Here's how the part is built. I have some questions about the finished solid (model axes, mm). A direction names the side the tool comes from. Coordinates: 2 decimals unless noted, no trailing zeros. Write each loop counter-clockwise with the first axis right and the second up, starting at its lowest first coordinate (ties: lowest second). Pieces come first, ordered by that corner, then holes.
Item 1: If we section it at B-B (y = 6): Please give me the cut outline in (x, z) (3 decimals), then the cut area to 3 significant figures.
Item 2: If we section it at A-A (x = -10.5): Please give me the cut outline in (y, z) (3 decimals), then the cut area to 3 significant figures.
Item 3: If we section it at C-C (z = 1): Please give me the cut outline in (x, y), then the cut area to 3 significant figures.
Item 4: I'm going to push flat-ended pins straight in: pin 1 Ø3 at (x, z) = (-9.5, -4.5) entering from +Y; pin 2 Ø2 at (x, z) = (5, 3.5) entering from -Y; pin 3 Ø1.2 at (x, y) = (6.5, -14) entering from +Z; pin 4 Ø0.8 at (x, z) = (-1.5, 4) entering from +Y. Where does each tip first touch, or does it pass through?
Item 5: We'd pull the mould along X, two halves only. Please class faces 4 (the face through (15.77, 0, 0)), 5 (the face through (3.493, 12.808, -4.081)), 6 (the face through (-6.15, 1, 8)): +X half, -X half, draft (parallel to the pull), parting line (faces both ways), or undercut.
Item 6: If we section it at D-D (z = 3.75): Please give me the cut outline in (x, y).
Item 7: For faces 1 (the face through (0, -12.7, 4)), 2 (the face through (3.283, 14.174, 4.078)), 3 (the face through (12.8, 0, 0)), which set-ups out of +Z, -Z, +X, -X, +Y, -Y let a thin tool reach every point of the face, with its end or its side?
Item 8: If I drill on line 1 (X direction, y = -7, z = -2.5); line 2 (Z direction, x = -10, y = 3) (3 decimals); line 3 (Y direction, x = -0.5, z = 3), over which ranges is the centre line in solid material (lowest first)?
from build123d import *

# Parameters (mm, degrees)
ESQUISSE1_W             = 31.54
ESQUISSE1_H             = 30.3
BOSS_EXTRU_1_DEPTH      = 6.71
ESQUISSE2_W             = 12.3
ESQUISSE2_H             = 15.3
BOSS_EXTRU_2_DEPTH      = 3.6
ESQUISSE9_W             = 25.6
ESQUISSE9_H             = 10.95
ENL_V_MAT_EXTRU_2_DEPTH = 36.680232623
BOSS_EXTRU_3_START      = -5.3
BOSS_EXTRU_3_DEPTH      = 6
ENL_V_MAT_EXTRU_1_DEPTH = 3.4
ESQUISSE5_W             = 16
ESQUISSE5_H             = 8.3
BOSS_EXTRU_4_DEPTH      = 0.8
BOSS_EXTRU_5_DEPTH      = 0.05
ESQUISSE7_W             = 4.9
ESQUISSE7_H             = 4.9
BOSS_EXTRU_6_DEPTH      = 1.8
ESQUISSE8_R             = 2.575
BOSS_EXTRU_7_DEPTH      = 3.55
ESQUISSE10_W            = 7
ESQUISSE10_H            = 3.3
BOSS_EXTRU_8_DEPTH      = 2.45
ESQUISSE11_W            = 3
ESQUISSE11_H            = 1.48
BOSS_EXTRU_9_DEPTH      = 0.3


with BuildPart() as part:
    # Esquisse1 → Boss.-Extru.1 (new, symmetric)
    with BuildSketch(Plane.XY):
        Rectangle(ESQUISSE1_W, ESQUISSE1_H)
    extrude(amount=BOSS_EXTRU_1_DEPTH, both=True)

    # Esquisse2 → Boss.-Extru.2 (add)
    with BuildSketch(Plane.XY.offset(6.71)):
        with Locations((0, 0.9)):
            Rectangle(ESQUISSE2_W, ESQUISSE2_H)
    extrude(amount=BOSS_EXTRU_2_DEPTH)

    # Esquisse9 → Enlèv. mat.-Extru.2 (cut, through all)
    with BuildSketch(Plane(origin=(0, 15.15, 0), x_dir=(1, 0, 0), z_dir=(0, 1, 0))):
        Rectangle(ESQUISSE9_W, ESQUISSE9_H)
    extrude(amount=-ENL_V_MAT_EXTRU_2_DEPTH, mode=Mode.SUBTRACT)

    # Esquisse3 → Boss.-Extru.3 (add)
    with BuildSketch(Plane(origin=(0, 15.15, 0), x_dir=(1, 0, 0), z_dir=(0, 1, 0)).offset(BOSS_EXTRU_3_START)):
        Polygon((-4, -2.56), (-3, -5.56), (3, -5.56), (4, -2.56), align=None)
    boss_extru_3 = extrude(amount=BOSS_EXTRU_3_DEPTH)

    # Esquisse4 → Enlèv. mat.-Extru.1 (cut)
    with BuildSketch(Plane(origin=(0, 15.85, 0), x_dir=(1, 0, 0), z_dir=(0, 1, 0))):
        Polygon((3.722514823, -2.76), (-3.722514823, -2.76), (-2.855848156, -5.36), (2.855848156, -5.36), align=None)
    enl_v_mat_extru_1 = extrude(amount=-ENL_V_MAT_EXTRU_1_DEPTH, mode=Mode.SUBTRACT)

    # Symétrie1: Boss.-Extru.3, Enlèv. mat.-Extru.1 across plane
    add(boss_extru_3.mirror(Plane.XY))
    add(enl_v_mat_extru_1.mirror(Plane.XY), mode=Mode.SUBTRACT)

    # Esquisse5 → Boss.-Extru.4 (add)
    with BuildSketch(Plane.XY.offset(6.71)):
        with Locations((0, -11)):
            Rectangle(ESQUISSE5_W, ESQUISSE5_H)
    extrude(amount=BOSS_EXTRU_4_DEPTH)

    # Esquisse6 → Boss.-Extru.5 (add)
    with BuildSketch(Plane.XY.offset(7.51)):
        Polygon((-6.865802853, -7.548465464), (-5.891959411, -7.548465464), (-5.891959411, -13.672228575), (-4.191256638, -13.672228575), (-4.191256638, -11.00969053), (-4.191256638, -10.559793746), (-1.795503566, -10.559793746), (-1.795503566, -11.00969053), (-1.795503566, -13.672228575), (-0.897751783, -13.672228575), (-0.897751783, -10.559793746), (0, -10.559793746), (1.676820822, -10.559793746), (1.676820822, -11.00969053), (1.676820822, -13.751215981), (5.361136535, -13.751215981), (5.361136535, -14.43345617), (1.676820822, -14.43345617), (0.989734758, -14.43345617), (0.989734758, -11.00969053), (0, -11.00969053), (0, -13.672228575), (0, -14.470915596), (-1.795503566, -14.470915596), (-2.368009826, -14.470915596), (-2.368009826, -11.00969053), (-3.468894756, -11.00969053), (-3.468894756, -13.672228575), (-3.468894756, -14.470915596), (-5.891959411, -14.470915596), (-6.865802853, -14.470915596), align=None)
    extrude(amount=BOSS_EXTRU_5_DEPTH)

    # Esquisse7 → Boss.-Extru.6 (add)
    with BuildSketch(Plane.XY.offset(6.71)):
        with Locations((-12.12, -11.5)):
            Rectangle(ESQUISSE7_W, ESQUISSE7_H)
    extrude(amount=BOSS_EXTRU_6_DEPTH)

    # Esquisse8 → Boss.-Extru.7 (add)
    with BuildSketch(Plane.XY.offset(6.71)):
        with Locations((11.77, -11.15)):
            Circle(ESQUISSE8_R)
    extrude(amount=BOSS_EXTRU_7_DEPTH)

    # Esquisse10 → Boss.-Extru.8 (add)
    with BuildSketch(Plane.XZ.offset(15.15)):
        with Locations((0, 3.86)):
            Rectangle(ESQUISSE10_W, ESQUISSE10_H)
        with Locations((-6.475, -3.86)):
            Rectangle(ESQUISSE10_W, ESQUISSE10_H)
        with Locations((6.475, -3.86)):
            Rectangle(ESQUISSE10_W, ESQUISSE10_H)
    extrude(amount=-BOSS_EXTRU_8_DEPTH)

    # Esquisse11 → Boss.-Extru.9 (add)
    with BuildSketch(Plane.XZ.offset(15.15)):
        with Locations((0, 3.8425)):
            Rectangle(ESQUISSE11_W, ESQUISSE11_H)
        with Locations((-6.475, -3.8425)):
            Rectangle(ESQUISSE11_W, ESQUISSE11_H)
        with Locations((6.475, -3.8425)):
            Rectangle(ESQUISSE11_W, ESQUISSE11_H)
    extrude(amount=BOSS_EXTRU_9_DEPTH)


solid = part.part
Answer list:
1. outline: (-15.77, -6.71) - (15.77, -6.71) - (15.77, 6.71) - (6.15, 6.71) - (6.15, 10.31) - (-6.15, 10.31) - (-6.15, 6.71) - (-15.77, 6.71) - close; hole (-12.8, -5.475) - (12.8, -5.475) - (12.8, 5.475) - (-12.8, 5.475) - close
1. area: 187 mm2
2. outline: (-15.15, -6.71) - (15.15, -6.71) - (15.15, -5.475) - (-15.15, -5.475) - close; (-15.15, 5.475) - (15.15, 5.475) - (15.15, 6.71) - (-9.05, 6.71) - (-9.05, 8.51) - (-13.95, 8.51) - (-13.95, 6.71) - (-15.15, 6.71) - close
2. area: 83.7 mm2
3. outline: (-15.77, -15.15) - (-12.8, -15.15) - (-12.8, 15.15) - (-15.77, 15.15) - close; (12.8, -15.15) - (15.77, -15.15) - (15.77, 15.15) - (12.8, 15.15) - close
3. area: 180 mm2
4. pin 1: stops at y = 15.15
4. pin 2: passes through
4. pin 3: stops at z = 7.51
4. pin 4: stops at y = 12.45
5. face 4: +X half
5. face 5: undercut
5. face 6: -X half
6. outline: (-15.77, -15.15) - (-12.8, -15.15) - (-12.8, 15.15) - (-15.77, 15.15) - close; (-3.6, 9.85) - (3.6, 9.85) - (3.6, 15.85) - (3.39, 15.85) - (3.39, 12.45) - (-3.39, 12.45) - (-3.39, 15.85) - (-3.6, 15.85) - close; (-3.5, -15.15) - (-1.5, -15.15) - (-1.5, -15.45) - (1.5, -15.45) - (1.5, -15.15) - (3.5, -15.15) - (3.5, -12.7) - (-3.5, -12.7) - close; (12.8, -15.15) - (15.77, -15.15) - (15.77, 15.15) - (12.8, 15.15) - close
7. face 1: none
7. face 2: +Y
7. face 3: +Y, -Y
8. line 1: x = -15.77 to -12.8, 12.8 to 15.77
8. line 2: z = -6.71 to -5.475, 5.475 to 6.71
8. line 3: y = -15.15 to -12.7, 9.85 to 12.45
